Geometry check sheet. Reference: the model listing, model coordinates, mm. A direction names the side the tool comes from. Coordinates: 2 decimals unless noted, no trailing zeros. Order: outer loops, then holes, each group sorted by start corner. A loop starts at its lowest first (then second) coordinate and runs counter-clockwise, first axis right, second up. Notation, with made-up numbers: M 53.5,15 L 63.5,15 A21 ccw 63.5,33 Z; hole C 34,-24.5 d10. An arc over 180 degrees is marked long. One line per item, written item: value. Start each with the question number.
1) Sectioned sample at C-C, the plane z = 3.5. Enter the section's corners in (x, y).
2) Sectioned sample at A-A, the plane y = 0. Enter the section's corners in (x, z), then the cut area to 3 significant figures.
3) Go/stop test with flat-tipped pins: P1, Ø1.5, axis at y = 3, z = 2.5, coming from the +X side; P2, Ø3, axis at y = 2, z = 1.5, coming from the -X side; P3, Ø4, axis at x = 0, y = 0, coming from the -Z side. Record where each tip stops, or that it passes through.
4) Access from +Z, -Z, +X, -X, +Y, -Y to the whole of each face (thin tool, end or side, straight path). Record for faces 1 (the cylindrical face through (-5.158, -3.955, 0.616)), 2 (the cylindrical face through (5, 0, 2)).
5) Draft check along Z on faces 3 (the flat face through (2, 5, 3.75)), 4 (the flat face through (3, -3, 0)), 5 (the flat face through (3, -3, 5)), 6 (the cylindrical face through (3.233, -1.341, 2.465)). Enter one of: pulls with the +Z half, pulls with the -Z half, needs draft (parallel to the pull), parting line crosses it, or undercut.
6) Thickness scan on L1, parallel to Y at x = 0, z = 2.3; L2, parallel to Z at x = -4, y = -4; L3, parallel to Y at x = 0, z = 3.85. Record the ranges inside material, lowest first. Write a range as from..to.
7) Sectioned sample at D-D, the plane y = -3.75. Enter the section's corners in (x, z), then the cut area to 3 significant figures.
```python
from build123d import *

# Parameters (mm, degrees)
ESQUISSE1_R        = 6.5
ESQUISSE1_R_2      = 3.5
BOSS_EXTRU_1_DEPTH = 5
ESQUISSE2_W        = 1.5
ESQUISSE2_H        = 2.5


with BuildPart() as part:
    # Esquisse1 → Boss.-Extru.1 (new body)
    with BuildSketch(Plane.XY):
        Circle(ESQUISSE1_R)
        Circle(ESQUISSE1_R_2, mode=Mode.SUBTRACT)
    extrude(amount=BOSS_EXTRU_1_DEPTH)

    # Esquisse2 → Enlèvement de matière-Révolution1 (revolve, cut)
    with BuildSketch(Plane(origin=(0, 0, 0), x_dir=(1, 0, 0), z_dir=(0, 1, 0)), mode=Mode.PRIVATE) as enl_vement_de_mati_re_r_volution1_sk:
        with Locations((5.75, -2.5)):
            Rectangle(ESQUISSE2_W, ESQUISSE2_H)
    revolve(enl_vement_de_mati_re_r_volution1_sk.sketch.rotate(Axis((0, 0, -1.624351993), (0, 0, 1)), 180), axis=Axis((0, 0, -1.624351993), (0, 0, 1)), mode=Mode.SUBTRACT)


solid = part.part
```
Final values:
1. outline: C 0,0 d10; hole C 0,0 d7
2. outline: M -6.5,0 L -3.5,0 L -3.5,5 L -6.5,5 L -6.5,3.75 L -5,3.75 L -5,1.25 L -6.5,1.25 Z; M 3.5,0 L 6.5,0 L 6.5,1.25 L 5,1.25 L 5,3.75 L 6.5,3.75 L 6.5,5 L 3.5,5 Z
2. area: 22.5 mm^2
3. P1: stops at x = 4.47
3. P2: stops at x = -6.48
3. P3: passes through
4. face 1: +Z, -Z
4. face 2: none
5. face 3: undercut
5. face 4: pulls with the -Z half
5. face 5: pulls with the +Z half
5. face 6: needs draft
6. L1: y = -5..-3.5, 3.5..5
6. L2: z = 0..1.25, 3.75..5
6. L3: y = -6.5..-3.5, 3.5..6.5
7. outline: M -5.31,0 L 5.31,0 L 5.31,1.25 L 3.31,1.25 L 3.31,3.75 L 5.31,3.75 L 5.31,5 L -5.31,5 L -5.31,3.75 L -3.31,3.75 L -3.31,1.25 L -5.31,1.25 Z
7. area: 43.1 mm^2
